Autodesk Inventor part; units mm, degrees
ref_plane "YZ Plane" through (0, 0, 0) normal (1, 0, 0) x (0, 1, 0)
ref_plane "XZ Plane" through (0, 0, 0) normal (0, 1, 0) x (-1, 0, 0)
ref_plane "XY Plane" through (0, 0, 0) normal (0, 0, 1) x (1, 0, 0)
sketch "Sketch1" plane through (0, 0, 0) normal (0, 1, 0) x (-1, 0, 0)
  line L0 (0, 0) -> (0, -600)
  line L1 (0, -600) -> (70, -600)
  line L2 (70, -600) -> (70, 0)
  line L3 (70, 0) -> (0, 0)
  line L4 (0, 0) -> (0, -300)
  line L5 (-3.2, -280) -> (-3.2, -320)
  line L6 (-3.2, -320) -> (0, -320)
  line L7 (-3.2, -280) -> (0, -280)
  line L8 (-3.2, -420) -> (0, -420)
  line L9 (-3.2, -420) -> (-3.2, -460)
  line L10 (-3.2, -460) -> (0, -460)
  line L11 (-3.2, -180) -> (0, -180)
  line L12 (-3.2, -180) -> (-3.2, -140)
  line L13 (-3.2, -140) -> (0, -140)
  line L14 (73.2, -280) -> (73.2, -320)
  line L15 (73.2, -320) -> (70, -320)
  line L16 (73.2, -280) -> (70, -280)
  line L17 (73.2, -420) -> (70, -420)
  line L18 (73.2, -420) -> (73.2, -460)
  line L19 (73.2, -460) -> (70, -460)
  line L20 (73.2, -180) -> (70, -180)
  line L21 (73.2, -180) -> (73.2, -140)
  line L22 (73.2, -140) -> (70, -140)
  dimension "d0" = 600
  dimension "d2" = 70
  dimension "d3" = 600
  dimension "d7" = 40
  dimension "d8" = 100
  dimension "d9" = 40
  dimension "d10" = 100
  dimension "d11" = 40
extrude "Extrusion1" add sketch "Sketch1" along normal blind 3.175
properties part number "Trebuchet V1 - Runway"
Read the model definition and answer for the solid it produces. Units are mm, in the model's axes. Coordinates: 2 decimals unless noted, no trailing zeros. Loops run counter-clockwise (first coordinate to the right, second up) from the corner with the lowest first, then second, coordinate; pieces in that order, holes last. Notation, with made-up numbers: (-14, 18) -> (31, 18) arc R23 cw to (31, 40) -> close; hole circle Ø4 at (48, 14). An arc over 180 degrees is marked (long way). Answer in a Markdown table with one row per item.
Item 1: A cutting plane is placed at A-A on y = 0.6. Determine the outline of the cut face in (x, z).
Returned:
| item | result |
|---|---|
| outline | (-73.2, -460) -> (-70, -460) -> (-70, -600) -> (0, -600) -> (0, -460) -> (3.2, -460) -> (3.2, -420) -> (0, -420) -> (0, -320) -> (3.2, -320) -> (3.2, -280) -> (0, -280) -> (0, -180) -> (3.2, -180) -> (3.2, -140) -> (0, -140) -> (0, 0) -> (-70, 0) -> (-70, -140) -> (-73.2, -140) -> (-73.2, -180) -> (-70, -180) -> (-70, -280) -> (-73.2, -280) -> (-73.2, -320) -> (-70, -320) -> (-70, -420) -> (-73.2, -420) -> close |
Item 2: Each of these flat-tipped pins is pushed along its axis until it touches: P1, Ø1.6, axis at x = -72, y = 2, coming from the -Z side; P2, Ø1, axis at y = 1.5, z = -206.5, coming from the -X side; P3, Ø1, axis at x = 1.5, y = 2, coming from the +Z side. Where does it stop, or does it pass through?
Returned:
| item | result |
|---|---|
| P1 | stops at z = -460 |
| P2 | stops at x = -70 |
| P3 | stops at z = -140 |
Item 3: A cutting plane is placed at B-B on z = -51.5. Determine the outline of the cut face in (x, y) (3 decimals).
Returned:
| item | result |
|---|---|
| outline | (-70, 0) -> (0, 0) -> (0, 3.175) -> (-70, 3.175) -> close |
Item 4: A straight line is drawn through the part: line 1 along X through (y, z) = (1.2, -49.5). Find the intervals that lie inside material, in ascending order. Write a range as [from, to].
Returned:
| item | result |
|---|---|
| line 1 | x = [-70, 0] |
